from build123d import *

# Parameters (mm, degrees)
F1_DEPTH = 18.9
F2_R     = 8.49999
F4_DEPTH = 0.4
F5_R     = 2.5
F6_DEPTH = 10
F7_R     = 2.5
F8_DEPTH = 25


# Not quite as in the source:
# - a fillet or chamfer is up to 0.001 mm smaller than in the source, because OpenCascade refuses the exact size


with BuildPart() as f1:
    # F0 (on Front) → F1 (new body)
    with BuildSketch(Plane.XZ):
        with BuildLine():
            ThreePointArc((-8.5, 0), (0, 8.5), (8.5, 0))
            Line((8.5, 0), (8.5, 29.3))
            Line((8.5, 29.3), (-8.5, 29.3))
            Line((-8.5, 29.3), (-8.5, 0))
        make_face()
        with BuildLine():
            Line((-8.5, 0), (8.5, 0))
            ThreePointArc((8.5, 0), (0, 8.5), (-8.5, 0))
        make_face()
        with BuildLine():
            ThreePointArc((-8.5, 0), (0, -8.5), (8.5, 0))
            Line((8.5, 0), (-8.5, 0))
        make_face()
    extrude(amount=F1_DEPTH)

    # F2 (radius 8.5 in the source; OpenCascade refuses exactly that, so slightly less here)
    f2_edges = [f1.edges().sort_by_distance(p)[0] for p in [
        (8.5, -18.9, 14.65),
    ]]
    fillet(f2_edges, radius=F2_R)

    # F3 (on face) → F4 (join)
    with BuildSketch(Plane.XY.offset(29.3)):
        with BuildLine():
            ThreePointArc((0, -18.9), (5.5861435714, -16.5861435714), (7.9, -11))
            ThreePointArc((7.9, -11), (-5.5861435714, -5.4138564286), (0, -18.9))
        make_face()
    extrude(amount=F4_DEPTH)

    # F5 (on face) → F6 (cut)
    with BuildSketch(Plane(origin=(0, 0, 0), x_dir=(-1, 0, 0), z_dir=(0, 1, 0))):
        with Locations((0, 20.5)):
            Circle(F5_R)
        with Locations((0, 1.5)):
            Circle(F5_R)
    extrude(amount=-F6_DEPTH, mode=Mode.SUBTRACT)

    # F7 (on face) → F8 (cut)
    with BuildSketch(Plane.XY.offset(29.7)):
        with Locations((0, -11)):
            Circle(F7_R)
    extrude(amount=-F8_DEPTH, mode=Mode.SUBTRACT)


solid = f1.part
Source: CAD feature listing. Evaluate the final solid. Frame: model axes, mm. A direction names the side the tool comes from. Give positions to 0.01 mm unless a question says otherwise; leave off trailing zeros. Order: outer loops, then holes, each group sorted by start corner. A loop starts at its lowest first (then second) coordinate and runs counter-clockwise, first axis right, second up. Notation, with made-up numbers: (-9.75, -2.5) -> (36.25, -2.5) arc R15 ccw to (36.25, 14.5) -> close; hole circle Ø10 at (-34.75, 48). An arc over 180 degrees is marked (long way). Use a Markdown table: item, result.
1) Mould query, pull axis X, two halves, no side actions, for faces 4 (the cylindrical face through (0, -5, 4)), 5 (the flat face through (8.5, -5, 14)), 6 (the flat face through (-1, -3, 29.3)). Classes: +X half, -X half, draft (parallel to the pull), parting line (faces both ways), or undercut.
Answer list:
| item | result |
|---|---|
| face 4 | undercut |
| face 5 | +X half |
| face 6 | draft |
2) Section query B-B, the plane y = -4.75. Return the cut outline in (x, z).
Answer list:
| item | result |
|---|---|
| outline | (-8.5, 0) arc R8.5 ccw to (8.5, 0) -> (8.5, 29.3) -> (4.83, 29.3) -> (4.83, 29.7) -> (-4.83, 29.7) -> (-4.83, 29.3) -> (-8.5, 29.3) -> close; hole circle Ø5 at (0, 1.5); hole circle Ø5 at (0, 20.5) |
3) Reachability of faces 1 (the cylindrical face through (0.54, -4.93, 18.06)), 2 (the cylindrical face through (-0.187, -5.127, -8.498)), 3 (the flat face through (0, -11, 4.7)) from +Z, -Z, +X, -X, +Y, -Y: full face, straight path, thin tool, end or side. Return the list, or none.
Answer list:
| item | result |
|---|---|
| face 1 | +Y |
| face 2 | -Z, +Y, -Y |
| face 3 | +Z |
4) Contact query for flat-ended pins moving along their axis: P1, Ø3, axis at y = -14, z = 6.5, coming from the -X side; P2, Ø2.5, axis at x = 0, z = 1, coming from the +Y side; P3, Ø6, axis at y = -16.5, z = 2.5, coming from the +X side. Output: stop coordinate, or through.
Answer list:
| item | result |
|---|---|
| P1 | x = -8.24 |
| P2 | y = -10 |
| P3 | x = 7.91 |
5) Section query D-D, the plane y = -8. Return the cut outline in (x, z).
Answer list:
| item | result |
|---|---|
| outline | (-8.5, 0) arc R8.5 ccw to (8.5, 0) -> (8.5, 29.3) -> (7.31, 29.3) -> (7.31, 29.7) -> (-7.31, 29.7) -> (-7.31, 29.3) -> (-8.5, 29.3) -> close; hole circle Ø5 at (0, 1.5); hole circle Ø5 at (0, 20.5) |
6) Ray query, line 1 along Z through (x, y) = (0, -6.75); line 2 along Z through (x, y) = (0, -3); line 3 along X through (y, z) = (-4.25, 20.5). Return the intervals inside material, ascending. Write a range as [from, to].
Answer list:
| item | result |
|---|---|
| line 1 | [-8.5, -1], [4, 18], [23, 29.7] |
| line 2 | [-8.5, -1], [4, 18], [23, 29.3] |
| line 3 | [-8.5, -2.5], [2.5, 8.5] |
